from build123d import *

# Parameters (mm, degrees)
EXTRUDE_1_DEPTH = 20


with BuildPart() as part:
    # 草图1 → 凸台-拉伸1 (new body)
    with BuildSketch(Plane(origin=(0, 0, 0), x_dir=(1, 0, 0), z_dir=(0, 1, 0))):
        Polygon((0, 40), (0, 0), (40, 0), (40, 4), (22.576549518, 4), (4, 24.728267981), (4, 40), align=None)
    extrude(amount=EXTRUDE_1_DEPTH)


solid = part.part
Could you check a few things on this model? Use its own coordinates, in mm. A direction names the side the tool comes from. Give positions to 0.01 mm unless a question says otherwise; leave off trailing zeros. Order: outer loops, then holes, each group sorted by start corner. A loop starts at its lowest first (then second) coordinate and runs counter-clockwise, first axis right, second up. Notation, with made-up numbers: (13.5, -16) -> (49.5, -16) arc R8 cw to (49.5, -10) -> close; hole circle Ø4 at (72, -3). An arc over 180 degrees is marked (long way). Answer in a Markdown table with one row per item. Add a question column.
Item 1: I'm going to push flat-ended pins straight in: P1, Ø1.5, axis at y = 4, z = -16, coming from the -X side; P2, Ø1.5, axis at y = 13.5, z = -17, coming from the +X side; P3, Ø8.5, axis at x = 29, y = 13, coming from the -Z side; P4, Ø8, axis at y = 15.5, z = -23, coming from the +X side. Where does each tip first touch, or does it pass through?
Item 2: Imagine slicing it at A-A (y = 14.25). List the corners of the cut face in (x, z) for me.
Item 3: Please list where these lines run through material, in increasing order: probe 1 along Z at (x, y) = (30.5, 2); probe 2 along X at (y, z) = (15, -29); probe 3 along X at (y, z) = (10, -23).
Item 4: Imagine slicing it at B-B (x = 35.5). List the corners of the cut face in (y, z) for me, and give its area (3 significant figures).
Item 5: Imagine slicing it at C-C (z = -34). List the corners of the cut face in (x, y) for me.
Item 6: For faces 1 (the flat face through (31, 10, -4)), 2 (the flat face through (20, 10, 0)), which set-ups out of +Z, -Z, +X, -X, +Y, -Y let a thin tool reach every point of the face, with its end or its side?
Result:
| question | item | result |
|---|---|---|
| 1 | P1 | x = 0 |
| 1 | P2 | x = 11.6 |
| 1 | P3 | z = -4 |
| 1 | P4 | x = 9.13 |
| 2 | outline | (0, -40) -> (4, -40) -> (4, -24.73) -> (22.58, -4) -> (40, -4) -> (40, 0) -> (0, 0) -> close |
| 3 | probe 1 | -4 to 0 |
| 3 | probe 2 | 0 to 4 |
| 3 | probe 3 | 0 to 5.55 |
| 4 | outline | (0, -4) -> (20, -4) -> (20, 0) -> (0, 0) -> close |
| 4 | area | 80.0 mm2 |
| 5 | outline | (0, 0) -> (4, 0) -> (4, 20) -> (0, 20) -> close |
| 6 | face 1 | -Z, +X, +Y, -Y |
| 6 | face 2 | +Z, +X, -X, +Y, -Y |
